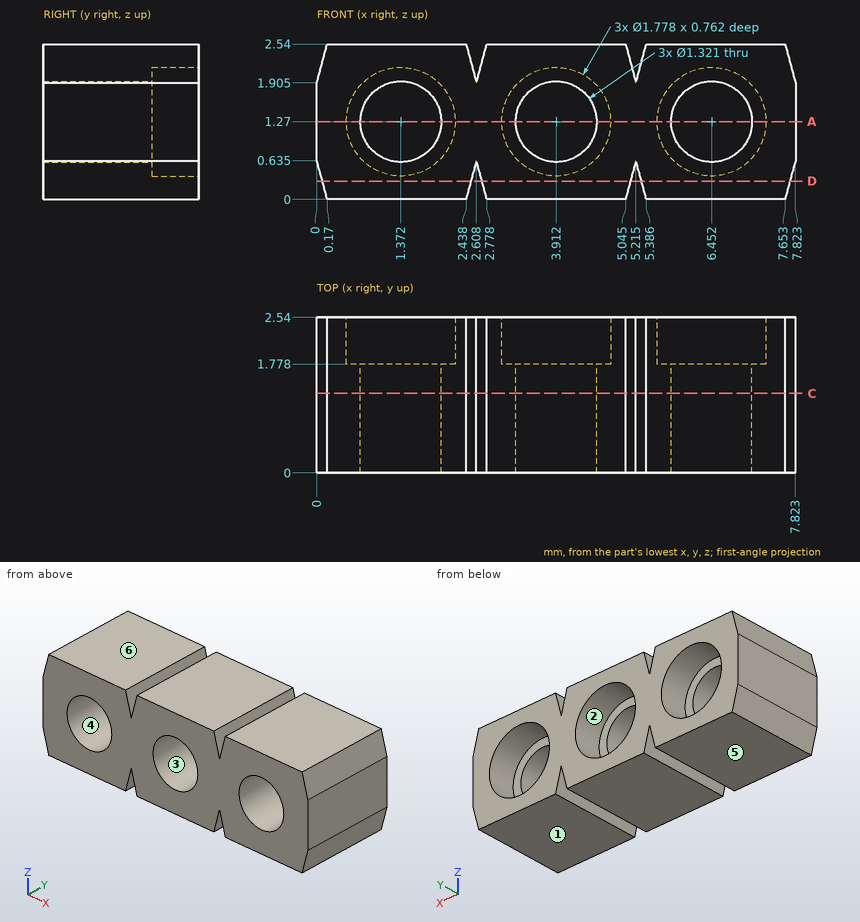
Source: three-view drawing plus pictorial views. Frame: mm from the lowest corner of the part. A direction names the side the tool comes from. Round coordinates to 2 decimals unless told otherwise and drop trailing zeros. Loops run counter-clockwise (first coordinate to the right, second up) from the corner with the lowest first, then second, coordinate; pieces in that order, holes last.
Q1. Section D-D, the plane z = 0.3. Return loops of the section in (x, y) (1 decimal), plus the area to 3 significant figures.
Q2. Mould query, pull axis Z, two halves, no side actions, for the marked faces 3, 4, 5 and 6. Classes: pulls with the +Z half, pulls with the -Z half, needs draft (parallel to the pull), parting line crosses it, or undercut.
Q3. Access query for the marked faces 1 and 2. Directions: +Z, -Z, +X, -X, +Y, -Y. A direction counts if a zero-diameter tool reaches every point of the face in a straight line with its end or side. Return the directions, or none.
Q4. Ray query, line 1 (X direction, y = 0.7, z = 1.27); line 2 (X direction, y = 1.1, z = 1.5); line 3 (X direction, y = 2.35, z = 0.3) (1 decimal). Return the intervals inside material, ascending.
Q5. First-contact query: P1, Ø1.1, axis at x = 6.45, z = 1.27, coming from the -Y side; P2, Ø0.5, axis at x = 6, z = 1.5, coming from the +Y side. Flat tips, straight axial feed; report the tip coordinate or a pass-through.
Q6. Section C-C, the plane y = 1.3. Return loops of the section in (x, z) (1 decimal).
Q7. Section A-A, the plane z = 1.27. Return loops of the section in (x, y).
Solutions:
1. outline: (0.1, 0) - (2.5, 0) - (2.5, 2.5) - (0.1, 2.5) - close; (2.7, 0) - (5.1, 0) - (5.1, 2.5) - (2.7, 2.5) - close; (5.3, 0) - (7.7, 0) - (7.7, 2.5) - (5.3, 2.5) - close
1. area: 18.5 mm2
2. face 3: undercut
2. face 4: undercut
2. face 5: pulls with the -Z half
2. face 6: pulls with the +Z half
3. face 1: -Z, +X, -X, +Y, -Y
3. face 2: +Y
4. line 1: x = 0 to 0.71, 2.03 to 3.25, 4.57 to 5.79, 7.11 to 7.82
4. line 2: x = 0 to 0.75, 1.99 to 3.29, 4.53 to 5.83, 7.07 to 7.82
4. line 3: x = 0.1 to 2.5, 2.7 to 5.1, 5.3 to 7.7
5. P1: passes through
5. P2: stops at y = 1.78
6. outline: (0, 0.6) - (0.2, 0) - (2.4, 0) - (2.6, 0.6) - (2.8, 0) - (5, 0) - (5.2, 0.6) - (5.4, 0) - (7.7, 0) - (7.8, 0.6) - (7.8, 1.9) - (7.7, 2.5) - (5.4, 2.5) - (5.2, 1.9) - (5, 2.5) - (2.8, 2.5) - (2.6, 1.9) - (2.4, 2.5) - (0.2, 2.5) - (0, 1.9) - close; hole circle Ø1.3 at (1.4, 1.3); hole circle Ø1.3 at (3.9, 1.3); hole circle Ø1.3 at (6.5, 1.3)
7. outline: (0, 0) - (0.71, 0) - (0.71, 1.78) - (0.48, 1.78) - (0.48, 2.54) - (0, 2.54) - close; (2.03, 0) - (3.25, 0) - (3.25, 1.78) - (3.02, 1.78) - (3.02, 2.54) - (2.26, 2.54) - (2.26, 1.78) - (2.03, 1.78) - close; (4.57, 0) - (5.79, 0) - (5.79, 1.78) - (5.56, 1.78) - (5.56, 2.54) - (4.8, 2.54) - (4.8, 1.78) - (4.57, 1.78) - close; (7.11, 0) - (7.82, 0) - (7.82, 2.54) - (7.34, 2.54) - (7.34, 1.78) - (7.11, 1.78) - close
